```python
from build123d import *

# Parameters (mm, degrees)
SKETCH1_R           = 99.25
SKETCH1_R_2         = 25.875
BOSS_EXTRUDE1_DEPTH = 3.7
FILLET1_R           = 1.85
SKETCH2_R           = 40
SKETCH2_R_2         = 25.875
BOSS_EXTRUDE2_DEPTH = 12
BOSS_EXTRUDE3_START = 28.6
SKETCH3_R           = 40
SKETCH3_R_2         = 35
BOSS_EXTRUDE3_DEPTH = 28.6


with BuildPart() as part:
    # Sketch1 → Boss-Extrude1 (new body)
    with BuildSketch(Plane(origin=(0, 0, 0), x_dir=(1, 0, 0), z_dir=(0, 1, 0))):
        with Locations(Location((0, 0, 0), (0, 0, 270))):
            Circle(SKETCH1_R)
        with Locations(Location((0, 0, 0), (0, 0, 270))):
            Circle(SKETCH1_R_2, mode=Mode.SUBTRACT)
    extrude(amount=BOSS_EXTRUDE1_DEPTH)

    # Fillet1
    fillet1_edges = [part.edges().sort_by_distance(p)[0] for p in [
        (0, 0, -99.25),
        (0, 3.7, -99.25),
    ]]
    fillet(fillet1_edges, radius=FILLET1_R - 0.0001)  # a hair under: the kernel refuses the full size

    # Sketch2 → Boss-Extrude2 (add)
    with BuildSketch(Plane(origin=(0, 3.7, 0), x_dir=(1, 0, 0), z_dir=(0, 1, 0))):
        with Locations(Location((0, 0, 0), (0, 0, 270))):
            Circle(SKETCH2_R)
        with Locations(Location((0, 0, 0), (0, 0, 270))):
            Circle(SKETCH2_R_2, mode=Mode.SUBTRACT)
    extrude(amount=BOSS_EXTRUDE2_DEPTH)


with BuildPart() as body_2:
    # Mirror2: mirrored copy
    add(part.part.mirror(Plane.ZX.offset(30)))


with BuildPart() as part_1:
    add(part.part)

    add(body_2.part)  # Boss-Extrude3 merges body 2
    # Sketch3 → Boss-Extrude3 (add)
    with BuildSketch(Plane.XZ.offset(-44.3).offset(BOSS_EXTRUDE3_START)):
        with Locations(Location((0, 0, 0), (0, 0, 90))):
            Circle(SKETCH3_R)
        with Locations(Location((0, 0, 0), (0, 0, 90))):
            Circle(SKETCH3_R_2, mode=Mode.SUBTRACT)
    extrude(amount=-BOSS_EXTRUDE3_DEPTH)


solid = part_1.part
```
Work out the finished part from the listing and answer in its coordinate system (mm). A direction names the side the tool comes from. Round coordinates to 2 decimals unless told otherwise and drop trailing zeros. Write each loop counter-clockwise with the first axis right and the second up, starting at its lowest first coordinate (ties: lowest second). Pieces come first, ordered by that corner, then holes.
1) A cutting plane is placed at C-C on y = 38. Determine the outline of the cut face in (x, z), and give its area (3 significant figures).
2) Which of the six approach directions +Z, -Z, +X, -X, +Y, -Y give full straight-line access (tool end or side, diameter ignored) to faces 1 (the face through (39.05, 29.63, -8.67)), 2 (the face through (7.77, 52.26, 24.68))?
3) Determine the mould class of faces 3 (the face through (1, 56.3, 42)), 4 (the face through (-20, 60, 20)), 5 (the face through (7.77, 7.74, 24.68)), 6 (the face through (-20, 0, 20)) for opening direction Y: pulls with the +Y half, pulls with the -Y half, needs draft (parallel to the pull), parting line crosses it, or undercut.
4) Flat-ended cylindrical pins translate along their axes: P1, Ø6, axis at y = 14, z = -12, coming from the +X side; P2, Ø12, axis at y = 43.5, z = -37, coming from the -X side; P3, Ø6, axis at y = 16, z = -13.5, coming from the +X side. Find the tip coordinate at first contact, or state that the pin passes through.
5) Consider probe 1 along Y at (x, z) = (-44, -38.5); probe 2 along X at (y, z) = (51, 0) (3 decimals); probe 3 along X at (y, z) = (33, 0). Determine where each line is inside the solid, lowest interval first.
Entries:
1. outline: circle Ø80 at (0, 0); hole circle Ø70 at (0, 0)
1. area: 1,180 mm2
2. face 1: none
2. face 2: +Y, -Y
3. face 3: undercut
3. face 4: pulls with the +Y half
3. face 5: needs draft
3. face 6: pulls with the -Y half
4. P1: stops at x = 38.97
4. P2: stops at x = -25.28
4. P3: stops at x = 38.6
5. probe 1: y = 0 to 3.7, 56.3 to 60
5. probe 2: x = -40 to -25.875, 25.875 to 40
5. probe 3: x = -40 to -35, 35 to 40
